Can you work these out from the model? Positions are in its coordinate system, mm. A direction names the side the tool comes from. Give positions to 0.01 mm unless a question says otherwise; leave off trailing zeros. Order: outer loops, then holes, each group sorted by start corner. A loop starts at its lowest first (then second) coordinate and runs counter-clockwise, first axis right, second up. Notation, with made-up numbers: (-21.5, 68) -> (9.5, 68) arc R13 cw to (9.5, 85) -> close; hole circle Ø11 at (76, -33). An arc over 180 degrees is marked (long way). Answer as CSV lines item,"result".
```python
from build123d import *

# Parameters (mm, degrees)
SKETCH_W       = 190
SKETCH_H       = 82
SKETCH_R       = 1.65
PAD_DEPTH      = 0.75
PAD_DEPTH_BACK = 0.75
POCKET_DEPTH   = 2.251


with BuildPart() as part:
    # Sketch → Pad (new body, two sides)
    with BuildSketch(Plane.XZ) as pad_sk:
        Rectangle(SKETCH_W, SKETCH_H)
        with Locations((90, 30)):
            Circle(SKETCH_R, mode=Mode.SUBTRACT)
        with Locations((90, 10)):
            Circle(SKETCH_R, mode=Mode.SUBTRACT)
        with Locations((90, -30)):
            Circle(SKETCH_R, mode=Mode.SUBTRACT)
        with Locations((90, -10)):
            Circle(SKETCH_R, mode=Mode.SUBTRACT)
        with Locations((-90, 30)):
            Circle(SKETCH_R, mode=Mode.SUBTRACT)
        with Locations((-90, 10)):
            Circle(SKETCH_R, mode=Mode.SUBTRACT)
        with Locations((-90, -30)):
            Circle(SKETCH_R, mode=Mode.SUBTRACT)
        with Locations((-90, -10)):
            Circle(SKETCH_R, mode=Mode.SUBTRACT)
    extrude(amount=PAD_DEPTH)
    extrude(pad_sk.sketch, amount=-PAD_DEPTH_BACK)

    # Sketch001 → Pocket (cut, through all)
    with BuildSketch(Plane.XZ.offset(1.5)):
        with BuildLine():
            ThreePointArc((-72.5, 12.5), (-85, 0), (-72.5, -12.5))
            Line((-72.5, -12.5), (72.5, -12.5))
            ThreePointArc((72.5, -12.5), (85, 0), (72.5, 12.5))
            Line((-72.5, 12.5), (72.5, 12.5))
        make_face()
    extrude(amount=-POCKET_DEPTH, mode=Mode.SUBTRACT)


solid = part.part
```
Item 1: We'd pull the mould along Z, two halves only. Please class faces 1 (the cylindrical face through (85, 0, 0)), 2 (the flat face through (-1, 0.75, 19)): released by +Z, released by -Z, zero draft, split by the parting line, or undercut.
Numbers:
face 1,"undercut"
face 2,"zero draft"
Item 2: Imagine slicing it at B-B, the plane z = 0. Please give me the cut outline in (x, y), then the cut area to 3 significant figures.
Numbers:
outline,"(-95, -0.75) -> (-85, -0.75) -> (-85, 0.75) -> (-95, 0.75) -> close; (85, -0.75) -> (95, -0.75) -> (95, 0.75) -> (85, 0.75) -> close"
area,"30.0 mm²"
Item 3: For pin 1 (3 mm diameter, centred on x = -90, z = -10, fed in from +Y), with a flat end and sliding along its axis, tell me the tip position at first contact or that it passes through.
Numbers:
pin 1,"passes through"
Item 4: Please list where these lines run through material, in increasing order: line 1 along Z through (x, y) = (90, -0.15); line 2 along Z through (x, y) = (15, -0.45); line 3 along X through (y, z) = (-0.3, -6.5).
Numbers:
line 1,"z = -41 to -31.65, -28.35 to -11.65, -8.35 to 8.35, 11.65 to 28.35, 31.65 to 41"
line 2,"z = -41 to -12.5, 12.5 to 41"
line 3,"x = -95 to -83.18, 83.18 to 95"
Item 5: Imagine slicing it at C-C, the plane y = -0.45. Give the number of separate pieces and of enclosed holes in the cut face, then the cut area to 3 significant figures.
Numbers:
separate pieces,"1"
enclosed holes,"9"
area,"11,400 mm²"
Item 6: Imagine slicing it at A-A, the plane x = -35. Please give me the cut outline in (y, z), then the cut area to 3 significant figures.
Numbers:
outline,"(-0.75, -41) -> (0.75, -41) -> (0.75, -12.5) -> (-0.75, -12.5) -> close; (-0.75, 12.5) -> (0.75, 12.5) -> (0.75, 41) -> (-0.75, 41) -> close"
area,"85.5 mm²"
Item 7: For faces 3 (the flat face through (-1, -0.75, 19)), 4 (the cylindrical face through (-85, 0, 0)), which set-ups out of +Z, -Z, +X, -X, +Y, -Y let a thin tool reach every point of the face, with its end or its side?
Numbers:
face 3,"+Z, -Z, +X, -X, -Y"
face 4,"+Y, -Y"
